The listing builds one solid part. Answer for the finished solid, in the listing's coordinates (mm). A direction names the side the tool comes from. Give positions to 0.01 mm unless a question says otherwise; leave off trailing zeros. Write each loop counter-clockwise with the first axis right and the second up, starting at its lowest first coordinate (ties: lowest second). Pieces come first, ordered by that corner, then holes. Notation, with made-up numbers: (14.25, -18) - (46.25, -18) arc R5 ccw to (46.25, -10) - close; hole circle Ø10 at (14.25, -18). An arc over 180 degrees is marked (long way). Write each question's results on one line, items separated by ' | '. Start each with the question number.
Q1. Section C-C (x = 3.81) is taken. Determine the outline of the cut face in (y, z), plus the area to 3 significant figures.
Q2. Section A-A (y = 2.25) is taken. Determine the outline of the cut face in (x, z), plus the area to 3 significant figures.
Q3. For faces 4 (the face through (1.288, 7.083, -5.486)), 5 (the face through (0.819, 0.811, -4.846)), 6 (the face through (4, 10.109, 5)), determine the directions among +Z, -Z, +X, -X, +Y, -Y from which every point of the face is accessible in a straight line to the end or side of a thin tool.
Q4. Section B-B (y = 7.25) is taken. State how many separate pieces and enclosed holes the cut face has, plus the area to 3 significant figures.
Q5. Section D-D (z = 1.75) is taken. Determine the outline of the cut face in (x, y).
Q6. Find the intervals of material crossed by probe 1 along Z at (x, y) = (2.25, 2); probe 2 along Z at (x, y) = (1.25, 4.25); probe 3 along Y at (x, z) = (-9, 5.75), in increasing order.
Q7. Flat-ended cylindrical pins translate along their axes: pin 1 Ø0.5 at (x, z) = (6.5, -5) entering from -Y; pin 2 Ø2 at (x, z) = (3, 4) entering from -Y; pin 3 Ø2 at (x, y) = (-1.5, 3) entering from +Z; pin 4 Ø1.3 at (y, z) = (3, -5) entering from -X. Find the tip coordinate at first contact, or state that the pin passes through.
Q8. For a pull along X with two mould halves and no side action, classify faces 1 (the face through (6.3, 1.6, -5.1)), 2 (the face through (-7.62, 3, 5)), 3 (the face through (-6.3, 10.109, 5.1)) as pulls with the +X half, pulls with the -X half, needs draft (parallel to the pull), parting line crosses it, or undercut.
```python
from build123d import *

# Parameters (mm, degrees)
BOSS_EXTRUDE1_DEPTH = 1.6002
SKETCH2_R           = 0.508
CUT_EXTRUDE1_DEPTH  = 13.80041562
LPATTERN1_COUNT     = 6
LPATTERN1_PITCH     = 2.54
SKETCH3_W           = 15.24
SKETCH3_H           = 2.54
SKETCH3_W_2         = 15.484150469
BOSS_EXTRUDE2_DEPTH = 2.54
SKETCH4_R           = 0.4064
BOSS_EXTRUDE3_DEPTH = 5.969
LPATTERN2_COUNT     = 6
LPATTERN2_PITCH     = 2.54


with BuildPart() as part:
    # Sketch1 → Boss-Extrude1 (new body)
    with BuildSketch(Plane(origin=(0, 0, 0), x_dir=(1, 0, 0), z_dir=(0, 1, 0))):
        with BuildLine():
            Line((-6.985, -7.62), (6.985, -7.62))
            ThreePointArc((6.985, -7.62), (9.23006403, -6.69006403), (10.16, -4.445))
            Line((10.16, -4.445), (10.16, 4.445))
            ThreePointArc((10.16, 4.445), (9.23006403, 6.69006403), (6.985, 7.62))
            Line((6.985, 7.62), (-6.985, 7.62))
            ThreePointArc((-6.985, 7.62), (-9.23006403, 6.69006403), (-10.16, 4.445))
            Line((-10.16, 4.445), (-10.16, -4.445))
            ThreePointArc((-10.16, -4.445), (-9.23006403, -6.69006403), (-6.985, -7.62))
        make_face()
    extrude(amount=BOSS_EXTRUDE1_DEPTH)

    # Sketch2 → Cut-Extrude1 (cut, symmetric)
    with BuildSketch(Plane(origin=(0, 1.6002, 0), x_dir=(1, 0, 0), z_dir=(0, 1, 0))):
        with Locations(Location((-6.35, 5.08, 0), (0, 0, 270))):
            Circle(SKETCH2_R)
        with Locations(Location((-6.35, -5.08, 0), (0, 0, 270))):
            Circle(SKETCH2_R)
    cut_extrude1 = extrude(amount=CUT_EXTRUDE1_DEPTH, both=True, mode=Mode.SUBTRACT)

    # LPattern1: Cut-Extrude1 ×6
    with Locations(*[(i * LPATTERN1_PITCH, 0, 0) for i in range(1, LPATTERN1_COUNT)]):
        add(cut_extrude1, mode=Mode.SUBTRACT)

    # Sketch3 → Boss-Extrude2 (add)
    with BuildSketch(Plane(origin=(0, 1.6002, 0), x_dir=(1, 0, 0), z_dir=(0, 1, 0))):
        with Locations((0, 5.08)):
            Rectangle(SKETCH3_W, SKETCH3_H)
        with Locations((0.122075235, -5.08)):
            Rectangle(SKETCH3_W_2, SKETCH3_H)
    extrude(amount=BOSS_EXTRUDE2_DEPTH)

    # Sketch4 → Boss-Extrude3 (add)
    with BuildSketch(Plane(origin=(0, 4.1402, 0), x_dir=(1, 0, 0), z_dir=(0, 1, 0))):
        with Locations(Location((-6.35, 5.08, 0), (0, 0, 270))):
            Circle(SKETCH4_R)
        with Locations(Location((-6.35, -5.08, 0), (0, 0, 270))):
            Circle(SKETCH4_R)
    boss_extrude3 = extrude(amount=BOSS_EXTRUDE3_DEPTH)

    # LPattern2: Boss-Extrude3 ×6
    with Locations(*[(i * LPATTERN2_PITCH, 0, 0) for i in range(1, LPATTERN2_COUNT)]):
        add(boss_extrude3)


solid = part.part
```
Answers below:
1) outline: (0, -7.62) - (1.6, -7.62) - (1.6, -6.35) - (4.14, -6.35) - (4.14, -5.49) - (10.11, -5.49) - (10.11, -4.67) - (4.14, -4.67) - (4.14, -3.81) - (1.6, -3.81) - (1.6, 3.81) - (4.14, 3.81) - (4.14, 4.67) - (10.11, 4.67) - (10.11, 5.49) - (4.14, 5.49) - (4.14, 6.35) - (1.6, 6.35) - (1.6, 7.62) - (0, 7.62) - (0, 5.59) - (1.6, 5.59) - (1.6, 4.57) - (0, 4.57) - (0, -4.57) - (1.6, -4.57) - (1.6, -5.59) - (0, -5.59) - close | area: 43.7 mm2
2) outline: (-7.62, -6.35) - (7.62, -6.35) - (7.62, -3.81) - (-7.62, -3.81) - close; (-7.62, 3.81) - (7.86, 3.81) - (7.86, 6.35) - (-7.62, 6.35) - close | area: 78.0 mm2
3) face 4: +Y | face 5: -Y | face 6: +Z, -Z, +X, -X, +Y
4) separate pieces: 12 | enclosed holes: 0 | area: 6.23 mm2
5) outline: (-10.16, 0) - (10.16, 0) - (10.16, 1.6) - (-10.16, 1.6) - close
6) probe 1: z = -6.35 to -3.81, 3.81 to 6.35 | probe 2: z = -5.49 to -4.67, 4.67 to 5.49 | probe 3: y = 0 to 1.6
7) pin 1: stops at y = 1.6 | pin 2: stops at y = 0 | pin 3: stops at z = 6.35 | pin 4: stops at x = -7.62
8) face 1: undercut | face 2: pulls with the -X half | face 3: needs draft
